Build history of the part. All positions in model axes, mm. A direction names the side the tool comes from. Round coordinates to 2 decimals unless told otherwise and drop trailing zeros. Write each loop counter-clockwise with the first axis right and the second up, starting at its lowest first coordinate (ties: lowest second). Pieces come first, ordered by that corner, then holes. Notation, with made-up numbers: (27, -4) -> (84, -4) arc R17 ccw to (84, 11) -> close; hole circle Ø9 at (-32.5, -5). An arc over 180 degrees is marked (long way). One line per question, with ' | ' between items.
from build123d import *

# Parameters (mm, degrees)
F1_DEPTH = 15.5


with BuildPart() as f1:
    # F0 (on Top) → F1 (new body)
    with BuildSketch(Plane.XY):
        with BuildLine():
            Line((0, 35), (0, 0))
            Line((0, 0), (90, 0))
            Line((90, 0), (90, 35))
            Line((90, 35), (90, 38.5))
            Line((90, 38.5), (90, 66.127198))
            Line((90, 66.127198), (77.497654, 66.127198))
            ThreePointArc((77.497654, 66.127198), (45, 80), (12.502346, 66.127198))
            Line((12.502346, 66.127198), (0, 66.127198))
            Line((0, 66.127198), (0, 38.5))
            Line((0, 38.5), (12.689011, 38.5))
            ThreePointArc((12.689011, 38.5), (45, 67.5), (77.310989, 38.5))
            ThreePointArc((77.310989, 38.5), (77.452713, 36.75255), (77.5, 35))
            ThreePointArc((77.5, 35), (45, 2.5), (12.5, 35))
            Line((12.5, 35), (0, 35))
        make_face()
    extrude(amount=F1_DEPTH)


solid = f1.part
(1) 3-axis set-ups, long thin cutter, end or side, ignore diameter. For faces 1 (the cylindrical face through (77.45, 36.78, 7.64)), 2 (the cylindrical face through (44.334, 67.493, 7.642)), 3 (the flat face through (6, 66.127, 8)): which of +Z, -Z, +X, -X, +Y, -Y reach the whole face in a straight line?
Calculated:
face 1: +Z, -Z, -X | face 2: +Z, -Z | face 3: +Z, -Z, -X, +Y
(2) Slice it at C-C (z = 2). Write the cut outline in (x, y), then the cut area to 3 significant figures.
Calculated:
outline: (0, 0) -> (90, 0) -> (90, 66.13) -> (77.5, 66.13) arc R45 ccw to (12.5, 66.13) -> (0, 66.13) -> (0, 38.5) -> (12.69, 38.5) arc R32.5 cw to (77.31, 38.5) arc R32.5 cw to (77.5, 35) arc R32.5 cw to (12.5, 35) -> (0, 35) -> close | area: 3,210 mm2
(3) Slice it at A-A (y = 63). Write the cut outline in (x, z).
Calculated:
outline: (0, 0) -> (28.5, 0) -> (28.5, 15.5) -> (0, 15.5) -> close; (61.5, 0) -> (90, 0) -> (90, 15.5) -> (61.5, 15.5) -> close
(4) Wall check: line 1 (Y direction, x = 9.5, z = 10.5); line 2 (Y direction, x = 54, z = 10.75); line 3 (X direction, y = 30, z = 12.5). Give the ranges that are in metal, low to high. Write a range as from..to.
Calculated:
line 1: 0..35, 38.5..66.13 | line 2: 0..3.77, 66.23..79.09 | line 3: 0..12.89, 77.11..90
(5) Drop flat-ended pins along their axis: pin 1 (6 mm diameter, centred on y = 71, z = 8, fed in from +X); pin 2 (1 mm diameter, centred on x = 79.5, z = 9, fed in from +Y); pin 3 (5 mm diameter, centred on x = 10.5, z = 13, fed in from +Y). Give the stop position or say it passes through.
Calculated:
pin 1: x = 75.59 | pin 2: y = 66.13 | pin 3: y = 66.64
(6) Mould opens along X. For faces 4 (the cylindrical face through (45.715, 2.508, 7.642)), 5 (the flat face through (34, 67, 15.5)), 6 (the flat face through (90, 33, 8)) say: pulls with the +X half, pulls with the -X half, needs draft (parallel to the pull), parting line crosses it, or undercut.
Calculated:
face 4: undercut | face 5: needs draft | face 6: pulls with the +X half
(7) Slice it at B-B (x = 73.5). Write the cut outline in (y, z).
Calculated:
outline: (0, 0) -> (19.38, 0) -> (19.38, 15.5) -> (0, 15.5) -> close; (50.62, 0) -> (69.82, 0) -> (69.82, 15.5) -> (50.62, 15.5) -> close
